```python
from build123d import *

# Parameters (mm, degrees)
F0_R     = 6.35
F1_DEPTH = 25.4


with BuildPart() as f1:
    # F0 (on Front) → F1 (new body)
    with BuildSketch(Plane.XZ):
        Polygon((-31.75, -1.27), (-31.75, -30.48), (31.75, -30.48), (31.75, 30.48), (-31.75, 30.48), (-31.75, 1.27), (3.81, 1.27), (8.171243, 0), (3.81, -1.27), align=None)
        with Locations((-19.05, -18.034)):
            Circle(F0_R, mode=Mode.SUBTRACT)
        with Locations((-19.05, 18.034)):
            Circle(F0_R, mode=Mode.SUBTRACT)
    extrude(amount=F1_DEPTH)


solid = f1.part
```
Input: part model. Units: mm. Frame: model coordinates. A direction names the side the tool comes from. Coordinates: 2 decimals unless noted, no trailing zeros. Loops run counter-clockwise (first coordinate to the right, second up) from the corner with the lowest first, then second, coordinate; pieces in that order, holes last. Notation, with made-up numbers: M 81.25,53.5 L 100.25,53.5 A26 ccw 100.25,67.5 Z; hole C -7.5,56.5 d10. An arc over 180 degrees is marked long. One line per item, written item: value.
(1) Section C-C (z = -15). Output: boundary loops of the cut face in (x, y), and give its area (3 significant figures).
Filled in:
outline: M -31.75,-25.4 L -24.63,-25.4 L -24.63,0 L -31.75,0 Z; M -13.47,-25.4 L 31.75,-25.4 L 31.75,0 L -13.47,0 Z
area: 1,330 mm^2
(2) Reachability of faces 1 (the flat face through (-14, -13, -1.27)), 2 (the cylindrical face through (-19.88, -12.52, -11.74)) from +Z, -Z, +X, -X, +Y, -Y: full face, straight path, thin tool, end or side. Return the list, or none.
Filled in:
face 1: -X, +Y, -Y
face 2: +Y, -Y
(3) Pull-direction query (X, two-part tool) for faces 3 (the cylindrical face through (-19.88, -12.52, 24.33)), 4 (the flat face through (-31.75, -13, -16)), 5 (the flat face through (0, -25.4, -6)), 6 (the flat face through (31.75, -13, 0)); classes: +X half, -X half, draft (parallel to the pull), parting line (faces both ways), or undercut.
Filled in:
face 3: undercut
face 4: -X half
face 5: draft
face 6: +X half
(4) Section A-A (x = -19.05). Output: boundary loops of the cut face in (y, z), and give its area (3 significant figures).
Filled in:
outline: M -25.4,-30.48 L 0,-30.48 L 0,-24.38 L -25.4,-24.38 Z; M -25.4,-11.68 L 0,-11.68 L 0,-1.27 L -25.4,-1.27 Z; M -25.4,1.27 L 0,1.27 L 0,11.68 L -25.4,11.68 Z; M -25.4,24.38 L 0,24.38 L 0,30.48 L -25.4,30.48 Z
area: 839 mm^2
(5) Section B-B (x = -8). Output: boundary loops of the cut face in (y, z), and give its area (3 significant figures).
Filled in:
outline: M -25.4,-30.48 L 0,-30.48 L 0,-1.27 L -25.4,-1.27 Z; M -25.4,1.27 L 0,1.27 L 0,30.48 L -25.4,30.48 Z
area: 1,480 mm^2
(6) Line query: line 1 along Z through (x, y) = (-19.05, -6.25); line 2 along Z through (x, y) = (-12, -17.5); line 3 along X through (y, z) = (-18.75, 21). Output: solid intervals per line, ascending. Write a range as from..to.
Filled in:
line 1: -30.48..-24.38, -11.68..-1.27, 1.27..11.68, 24.38..30.48
line 2: -30.48..-1.27, 1.27..30.48
line 3: -31.75..-24.66, -13.44..31.75
(7) Section D-D (y = -10.75). Output: boundary loops of the cut face in (x, z), and give its area (3 significant figures).
Filled in:
outline: M -31.75,-30.48 L 31.75,-30.48 L 31.75,30.48 L -31.75,30.48 L -31.75,1.27 L 3.81,1.27 L 8.17,0 L 3.81,-1.27 L -31.75,-1.27 Z; hole C -19.05,-18.03 d12.7; hole C -19.05,18.03 d12.7
area: 3,520 mm^2
(8) Pin query (flat end, axial travel): pin 1 (14.5 mm diameter, centred on x = -19.05, z = 18.034, fed in from +Y). Return the tip coordinate at first contact, or that it passes through.
Filled in:
pin 1: y = 0
